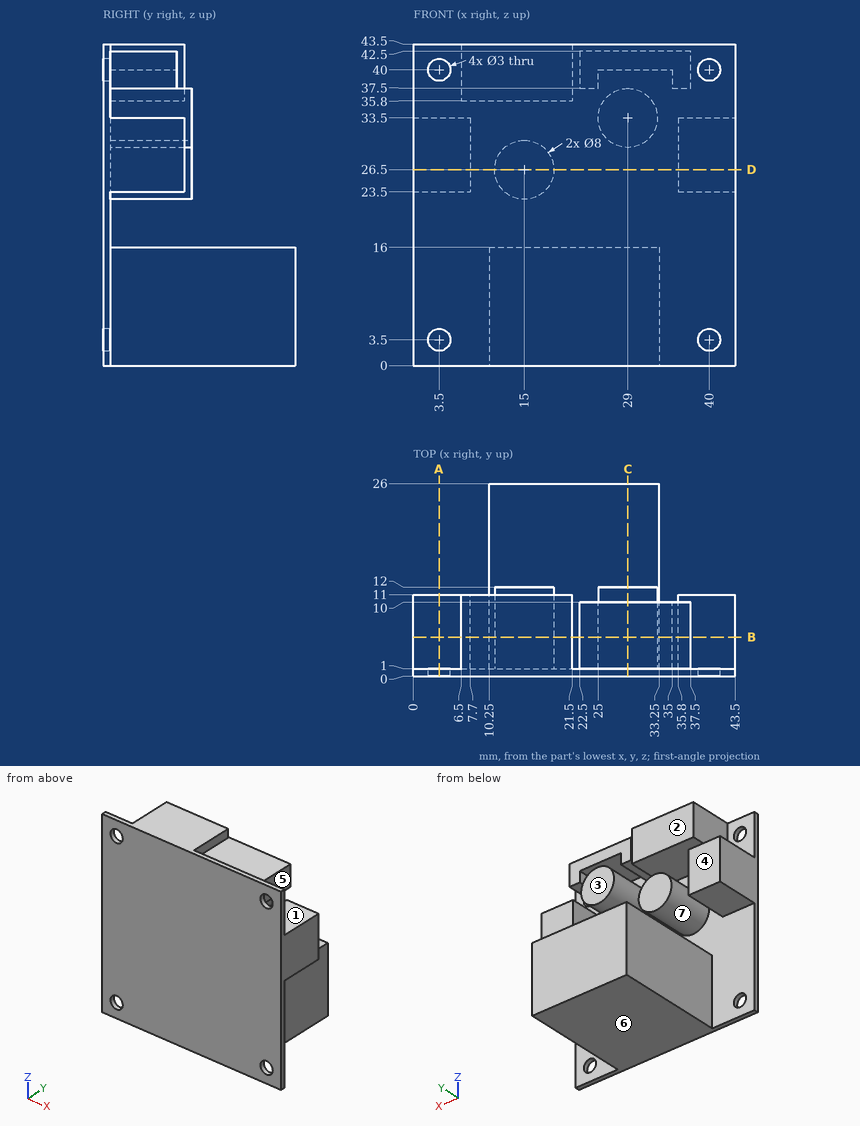
Geometry check sheet. Reference: drawing and pictorial views, mm from the part's lowest x, y, z. A direction names the side the tool comes from. Coordinates: 2 decimals unless noted, no trailing zeros. Loops run counter-clockwise (first coordinate to the right, second up) from the corner with the lowest first, then second, coordinate; pieces in that order, holes last.
1) Gauge pin test, flat ends, axial feed: pin 1 (5 mm diameter, centred on y = 10.5, z = 36.5, fed in from -X); pin 2 (11 mm diameter, centred on y = 4.5, z = 29, fed in from -X); pin 3 (8.5 mm diameter, centred on x = 38.5, y = 8, fed in from -Z); pin 4 (1.5 mm diameter, centred on x = 30, z = 21, fed in from +Y). Record the tip position at first contact, or that the pin passes through.
2) Sectioned sample at A-A (x = 3.5). Record the boundary of the cut face in (y, z), and give its area (4 significant figures).
3) Release check for a two-part mould opening along X. For the marked faces 5, 6 and 7 record: released by +X, released by -X, zero draft, split by the parting line, or undercut.
4) Access from +Z, -Z, +X, -X, +Y, -Y to the whole of each face (thin tool, end or side, straight path). Record for the marked faces 1, 2, 3 and 4.
5) Sectioned sample at C-C (x = 29). Record the boundary of the cut face in (y, z).
6) Sectioned sample at D-D (z = 26.5). Record the boundary of the cut face in (x, y), and give its area (4 significant figures).
7) Sectioned sample at B-B (y = 5.25). Record the boundary of the cut face in (x, z).
8) Material ranges on probe 1 along X at (y, z) = (0.7, 40); probe 2 along X at (y, z) = (6, 25.5); probe 3 along Z at (x, y) = (27, 4.5), recorded low to high.
Check sheet entries:
1. pin 1: stops at x = 6.5
1. pin 2: stops at x = 0
1. pin 3: stops at z = 23.5
1. pin 4: stops at y = 1
2. outline: (0, 0) - (1, 0) - (1, 2) - (0, 2) - close; (0, 5) - (1, 5) - (1, 23.5) - (11, 23.5) - (11, 33.5) - (1, 33.5) - (1, 38.5) - (0, 38.5) - close; (0, 41.5) - (1, 41.5) - (1, 43.5) - (0, 43.5) - close
2. area: 137.5 mm2
3. face 5: released by +X
3. face 6: zero draft
3. face 7: undercut
4. face 1: +X, +Y
4. face 2: +Z, -X, +Y
4. face 3: +Z, +X, -X, +Y
4. face 4: +Z, -Z, -X, +Y
5. outline: (0, 0) - (26, 0) - (26, 16) - (1, 16) - (1, 29.5) - (12, 29.5) - (12, 37.5) - (1, 37.5) - (1, 40) - (10, 40) - (10, 42.5) - (1, 42.5) - (1, 43.5) - (0, 43.5) - close
6. outline: (0, 0) - (43.5, 0) - (43.5, 11) - (35.8, 11) - (35.8, 1) - (19, 1) - (19, 12) - (11, 12) - (11, 1) - (7.7, 1) - (7.7, 11) - (0, 11) - close
6. area: 285.5 mm2
7. outline: (0, 23.5) - (7.7, 23.5) - (7.7, 33.5) - (0, 33.5) - close; (6.5, 35.8) - (21.5, 35.8) - (21.5, 43.5) - (6.5, 43.5) - close; (10.25, 0) - (33.25, 0) - (33.25, 16) - (10.25, 16) - close; circle Ø8 at (15, 26.5); (22.5, 37.5) - (25, 37.5) - (25, 40) - (35, 40) - (35, 37.5) - (37.5, 37.5) - (37.5, 42.5) - (22.5, 42.5) - close; circle Ø8 at (29, 33.5); (35.8, 23.5) - (43.5, 23.5) - (43.5, 33.5) - (35.8, 33.5) - close
8. probe 1: x = 0 to 2, 5 to 38.5, 41.5 to 43.5
8. probe 2: x = 0 to 7.7, 11.13 to 18.87, 35.8 to 43.5
8. probe 3: z = 0 to 16, 30.04 to 36.96, 40 to 42.5
